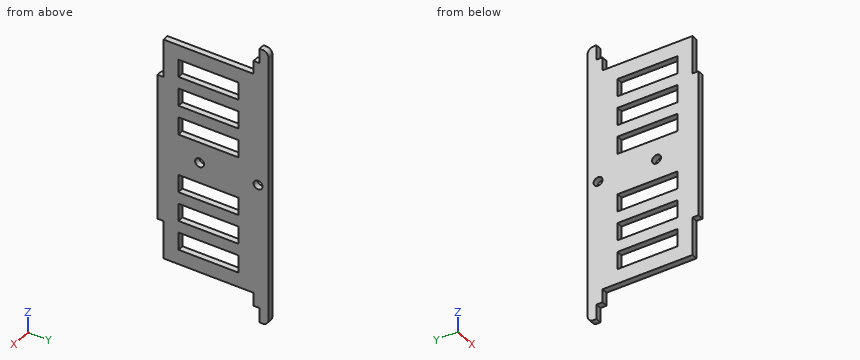
```python
from build123d import *

# Parameters (mm, degrees)
SKETCH1_R           = 1.5
SKETCH1_W           = 6
SKETCH1_H           = 20
BOSS_EXTRUDE1_DEPTH = 2
FILLET2_R           = 2


with BuildPart() as part:
    # Sketch1 → Boss-Extrude1 (new body)
    with BuildSketch(Plane(origin=(0, 0, 0), x_dir=(0, 0, -1), z_dir=(1, 0, 0))):
        Polygon((-25, -15), (-25, -17), (25, -17), (25, -15), (38, -15), (38, 15), (42.5, 15), (42.5, 17), (47.5, 17), (47.5, 20), (-47.5, 20), (-47.5, 17), (-42.5, 17), (-42.5, 15), (-38, 15), (-38, -15), align=None)
        with Locations((0, 16.5)):
            Circle(SKETCH1_R, mode=Mode.SUBTRACT)
        with Locations((0, -3)):
            Circle(SKETCH1_R, mode=Mode.SUBTRACT)
        with Locations((20, 0)):
            Rectangle(SKETCH1_W, SKETCH1_H, mode=Mode.SUBTRACT)
        with Locations((30, 0)):
            Rectangle(SKETCH1_W, SKETCH1_H, mode=Mode.SUBTRACT)
        with Locations((10, 0)):
            Rectangle(SKETCH1_W, SKETCH1_H, mode=Mode.SUBTRACT)
        with Locations((-10, 0)):
            Rectangle(SKETCH1_W, SKETCH1_H, mode=Mode.SUBTRACT)
        with Locations((-20, 0)):
            Rectangle(SKETCH1_W, SKETCH1_H, mode=Mode.SUBTRACT)
        with Locations((-30, 0)):
            Rectangle(SKETCH1_W, SKETCH1_H, mode=Mode.SUBTRACT)
    extrude(amount=BOSS_EXTRUDE1_DEPTH)

    # Fillet2
    fillet2_edges = [part.edges().sort_by_distance(p)[0] for p in [
        (1, 20, 47.5),
        (1, 20, -47.5),
    ]]
    fillet(fillet2_edges, radius=FILLET2_R)


solid = part.part
```
Here's how the part is built. I have some questions about the finished solid (model axes, mm). Coordinates: 2 decimals unless noted, no trailing zeros. Loops run counter-clockwise (first coordinate to the right, second up) from the corner with the lowest first, then second, coordinate; pieces in that order, holes last. Notation, with made-up numbers: (27, 11) -> (74, 11) arc R14 cw to (74, 30) -> close; hole circle Ø3 at (-10.5, 14). An arc over 180 degrees is marked (long way). Return JSON: item names as keys, results as strings.
1) Will these pins go through, and if not, where does the flat tip stop? pin 1 (0.6 mm diameter, centred on x = 1.5, y = -5, fed in from +Z); pin 2 (1 mm diameter, centred on x = 1, y = 0.5, fed in from -Z); pin 3 (1 mm diameter, centred on x = 1.5, y = -16, fed in from +Z).
Results below:
{"pin 1": "z = 38", "pin 2": "z = -38", "pin 3": "z = 25"}
2) If we section it at B-B, the plane y = -7: Write out the boundary of the cut face in (x, z), then the cut area to 3 significant figures.
Results below:
{"outline": "(0, -38) -> (2, -38) -> (2, -33) -> (0, -33) -> close; (0, -27) -> (2, -27) -> (2, -23) -> (0, -23) -> close; (0, -17) -> (2, -17) -> (2, -13) -> (0, -13) -> close; (0, -7) -> (2, -7) -> (2, 7) -> (0, 7) -> close; (0, 13) -> (2, 13) -> (2, 17) -> (0, 17) -> close; (0, 23) -> (2, 23) -> (2, 27) -> (0, 27) -> close; (0, 33) -> (2, 33) -> (2, 38) -> (0, 38) -> close", "area": "80.0 mm²"}
3) If we section it at D-D, the plane y = -3: Count the separate pieces of the cut face and the enclosed holes in it, then the cut area to 3 significant figures.
Results below:
{"separate pieces": "8", "enclosed holes": "0", "area": "74.0 mm²"}
4) If we section it at A-A, the plane z = 0: Write out the boundary of the cut face in (x, y), then the cut area to 3 significant figures.
Results below:
{"outline": "(0, -17) -> (2, -17) -> (2, -4.5) -> (0, -4.5) -> close; (0, -1.5) -> (2, -1.5) -> (2, 15) -> (0, 15) -> close; (0, 18) -> (2, 18) -> (2, 20) -> (0, 20) -> close", "area": "62.0 mm²"}
5) If we section it at C-C, the plane z = 12: Write out the boundary of the cut face in (x, y).
Results below:
{"outline": "(0, -17) -> (2, -17) -> (2, -10) -> (0, -10) -> close; (0, 10) -> (2, 10) -> (2, 20) -> (0, 20) -> close"}
6) I need wall thicknesses on line 1 (Y direction, x = 0.95, z = 0); line 2 (Y direction, x = 0.85, z = 29); line 3 (Y direction, x = 0.35, z = -12). Which ranges of each line are inside material? Lowest first, please. Write a range as from..to.
Results below:
{"line 1": "-17..-4.5, -1.5..15, 18..20", "line 2": "-15..-10, 10..20", "line 3": "-17..-10, 10..20"}
